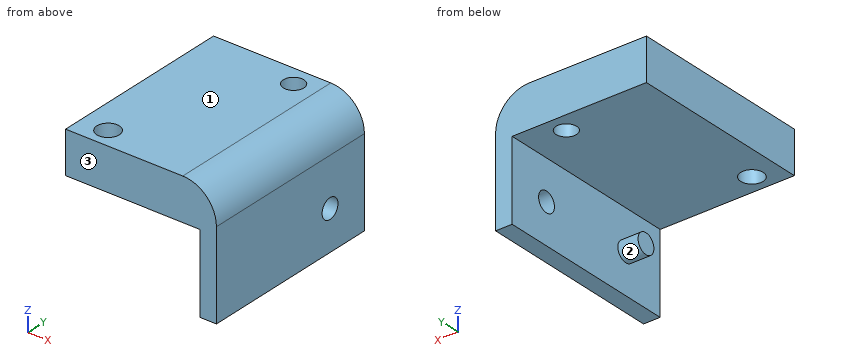
```python
from build123d import *

# Parameters (mm, degrees)
BOSS_EXTRUDE1_DEPTH = 27.9999948
SKETCH2_R           = 1.5
CUT_EXTRUDE1_DEPTH  = 3.5
SKETCH3_R           = 1.55
SKETCH3_R_2         = 1.7
CUT_EXTRUDE2_DEPTH  = 19.35
FILLET1_R           = 5.08
SKETCH2_3_R         = 1.5
BOSS_EXTRUDE2_DEPTH = 3.048


with BuildPart() as part:
    # Sketch1 → Boss-Extrude1 (new body)
    with BuildSketch(Plane(origin=(0, 0, 0), x_dir=(1, 0, 0), z_dir=(0, 1, 0))):
        Polygon((0, 18.35), (0, 0), (-22.7671934, 0), (-22.7671934, 6.35), (-2.5, 6.35), (-2.5, 18.35), align=None)
    extrude(amount=BOSS_EXTRUDE1_DEPTH)

    # Sketch2 → Cut-Extrude1 (cut, through all)
    with BuildSketch(Plane.ZY.offset(2.5)):
        with Locations((-12.35, 21.4999951)):
            Circle(SKETCH2_R)
    extrude(amount=-CUT_EXTRUDE1_DEPTH, mode=Mode.SUBTRACT)

    # Sketch3 → Cut-Extrude2 (cut, through all)
    with BuildSketch(Plane.XY):
        with Locations((-8.368, 25.0999974)):
            Circle(SKETCH3_R)
        with Locations((-18.668, 2.8999974)):
            Circle(SKETCH3_R_2)
    extrude(amount=-CUT_EXTRUDE2_DEPTH, mode=Mode.SUBTRACT)

    # Fillet1
    fillet1_edges = [part.edges().sort_by_distance(p)[0] for p in [
        (0, 13.9999974, 0),
    ]]
    fillet(fillet1_edges, radius=FILLET1_R)

    # Sketch2<3> → Boss-Extrude2 (add)
    with BuildSketch(Plane.ZY.offset(2.5)):
        with Locations((-12.35, 6.4999997)):
            Circle(SKETCH2_3_R)
    extrude(amount=BOSS_EXTRUDE2_DEPTH)


solid = part.part
```
Read the model definition and answer for the solid it produces. Units are mm, in the model's axes. Face numbers are marked on the shaded views. Round coordinates to 2 decimals unless told otherwise and drop trailing zeros. Write each loop counter-clockwise with the first axis right and the second up, starting at its lowest first coordinate (ties: lowest second). Pieces come first, ordered by that corner, then holes. Notation, with made-up numbers: (-19, 79) - (29, 79) arc R11 ccw to (29, 84) - close; hole circle Ø7 at (2, 52). An arc over 180 degrees is marked (long way). One line per item, written item: value.
Q1. Each of these flat-tipped pins is pushed along its axis until it touches: P1, Ø3, axis at x = -8.37, y = 25.1, coming from the -Z side; P2, Ø2.5, axis at y = 7, z = -13, coming from the -X side; P3, Ø2, axis at x = -5, y = 16.5, coming from the -Z side. Where does it stop, or does it pass through?
The answers:
P1: passes through
P2: stops at x = -5.55
P3: stops at z = -6.35
Q2. Find section A-A (z = -12.35). Determine the outline of the cut face in (x, y).
The answers:
outline: (-5.55, 5) - (-2.5, 5) - (-2.5, 0) - (0, 0) - (0, 20) - (-2.5, 20) - (-2.5, 8) - (-5.55, 8) - close; (-2.5, 23) - (0, 23) - (0, 28) - (-2.5, 28) - close
Q3. For a pull along Z with two mould halves and no side action, classify the marked faces 1, 2 and 3 as pulls with the +Z half, pulls with the -Z half, needs draft (parallel to the pull), parting line crosses it, or undercut.
The answers:
face 1: pulls with the +Z half
face 2: undercut
face 3: needs draft
Q4. Straight lines are drawn through the part: line 1 (Y direction, x = -1.4, z = -12.35); line 2 (Z direction, x = -5.5, y = 9.25); line 3 (X direction, y = 8.5, z = -12.5). For each, find the intervals that lie inside material, in ascending order. Write a range as from..to.
The answers:
line 1: y = 0..20, 23..28
line 2: z = -6.35..0
line 3: x = -2.5..0
Q5. Find section D-D (z = -4). Determine the outline of the cut face in (x, y), and give its area (3 significant figures).
The answers:
outline: (-22.77, 0) - (-0.12, 0) - (-0.12, 28) - (-22.77, 28) - close; hole circle Ø3.4 at (-18.67, 2.9); hole circle Ø3.1 at (-8.37, 25.1)
area: 618 mm2
Q6. Find section C-C (y = 17.5). Determine the outline of the cut face in (x, z).
The answers:
outline: (-22.77, -6.35) - (-2.5, -6.35) - (-2.5, -18.35) - (0, -18.35) - (0, -5.08) arc R5.08 ccw to (-5.08, 0) - (-22.77, 0) - close
Q7. Find section B-B (x = -19.75). Determine the outline of the cut face in (y, z).
The answers:
outline: (0, -6.35) - (1.59, -6.35) - (1.59, 0) - (0, 0) - close; (4.21, -6.35) - (28, -6.35) - (28, 0) - (4.21, 0) - close
